from build123d import *

# Parameters (mm, degrees)
F0_W     = 60
F0_H     = 100
F1_DEPTH = 600
F2_R     = 20
F4_D     = 50


with BuildPart() as f1:
    # F0 (on Top) → F1 (new body)
    with BuildSketch(Plane.XY):
        with Locations((0.74253, 27.593936)):
            Rectangle(F0_W, F0_H)
    extrude(amount=F1_DEPTH)

    # F2
    f2_edges = [f1.edges().sort_by_distance(p)[0] for p in [
        (-29.25747, -22.406064, 300),
        (30.74253, -22.406064, 300),
        (30.74253, 77.593936, 300),
        (-29.25747, 77.593936, 300),
    ]]
    fillet(f2_edges, radius=F2_R)

    # F4 (through all)
    with Locations(Plane.YZ.offset(30.74253)):
        with Locations((27.593936, 550), (25.096449, 50)):
            Hole(F4_D / 2)


solid = f1.part
The model under review builds one solid part; all positions refer to its coordinate system, in mm. Give positions to 0.01 mm unless a question says otherwise; leave off trailing zeros. Order: outer loops, then holes, each group sorted by start corner. A loop starts at its lowest first (then second) coordinate and runs counter-clockwise, first axis right, second up. Notation, with made-up numbers: (64.25, -23.5) -> (107.25, -23.5) arc R9 ccw to (107.25, -14.5) -> close; hole circle Ø4 at (83.25, 13). An arc over 180 degrees is marked (long way). Write item = value, one per line. Start each with the question number.
(1) Take a section at C-C (z = 374). Write out the cut boundary in (x, y).
(2) For pin 1 Ø3 at (y, z) = (63, 535) entering from +X; pin 2 Ø1 at (x, z) = (19.5, 219.5) entering from -Y; pin 3 Ø1 at (x, z) = (13.5, 396) entering from +Y, all flat-tipped, find the tip position at first contact; note any pin that passes through.
(3) Take a section at B-B (x = 2). Write out the cut boundary in (y, z), plus the area to 3 significant figures.
(4) Draft analysis for pull direction Y (two halves, no side actions). For faces 1 (the cylindrical face through (0.323, 14.154, 571.08)), 2 (the flat face through (0, 28, 0)), 3 (the flat face through (1, 77.594, 296)), state which applies: +Y half, -Y half, draft (parallel to the pull), parting line (faces both ways), or undercut.
(5) For L1, parallel to Z at x = -15, y = 40; L2, parallel to Z at x = 22, y = 34.5; L3, parallel to Y at x = 11.5, z = 41, list the stretches that pass through material, from the lowest coordinate up. Write a range as from..to.
(6) Take a section at D-D (z = 56). Write out the cut boundary in (x, y), plus the area to 3 significant figures.
(7) Take a section at A-A (z = 550). Write out the cut boundary in (x, y), plus the area to 3 significant figures.
Returned:
q1.outline = (-29.26, -2.41) arc R20 ccw to (-9.26, -22.41) -> (10.74, -22.41) arc R20 ccw to (30.74, -2.41) -> (30.74, 57.59) arc R20 ccw to (10.74, 77.59) -> (-9.26, 77.59) arc R20 ccw to (-29.26, 57.59) -> close
q2.pin_1 = 30.36
q2.pin_2 = -20.62
q2.pin_3 = 77.47
q3.outline = (-22.41, 0) -> (77.59, 0) -> (77.59, 600) -> (-22.41, 600) -> close; hole circle Ø50 at (25.1, 50); hole circle Ø50 at (27.59, 550)
q3.area = 56,100 mm²
q4.face_1 = undercut
q4.face_2 = draft
q4.face_3 = +Y half
q5.L1 = 0..29.93, 70.07..528.3, 571.7..600
q5.L2 = 0..26.84, 73.16..525.97, 574.03..600
q5.L3 = -22.39..1.77, 48.42..77.58
q6.outline = (-29.26, -2.41) arc R20 ccw to (-9.26, -22.41) -> (10.74, -22.41) arc R20 ccw to (30.74, -2.41) -> (30.74, 0.83) -> (-29.26, 0.83) -> close; (-29.26, 49.37) -> (30.74, 49.37) -> (30.74, 57.59) arc R20 ccw to (10.74, 77.59) -> (-9.26, 77.59) arc R20 ccw to (-29.26, 57.59) -> close
q6.area = 2,740 mm²
q7.outline = (-29.26, -2.41) arc R20 ccw to (-9.26, -22.41) -> (10.74, -22.41) arc R20 ccw to (30.74, -2.41) -> (30.74, 2.59) -> (-29.26, 2.59) -> close; (-29.26, 52.59) -> (30.74, 52.59) -> (30.74, 57.59) arc R20 ccw to (10.74, 77.59) -> (-9.26, 77.59) arc R20 ccw to (-29.26, 57.59) -> close
q7.area = 2,660 mm²
